Input: dimensioned drawing with shaded views. Units: mm. Origin: part minimum x, y, z. Round coordinates to 2 decimals unless told otherwise and drop trailing zeros. Loops run counter-clockwise (first coordinate to the right, second up) from the corner with the lowest first, then second, coordinate; pieces in that order, holes last. Notation, with made-up numbers: M 21.5,64 L 49.5,64 A21 cw 49.5,101 Z; hole C 65,-36 d9. An arc over 180 degrees is marked long. Write each question's results on one line, items separated by ' | '. Start each with the question number.
1. Section C-C on x = 2.25. Output: boundary loops of the cut face in (y, z), and give its area (3 significant figures).
2. Section B-B on y = 24.5. Output: boundary loops of the cut face in (x, z), and give its area (3 significant figures).
3. Draft query along X for the marked faces 1, 2, 3 and 4. Return one class per face: released by +X, released by -X, zero draft, split by the parting line, or undercut.
4. Contact query for flat-ended pins moving along their axis: pin 1 Ø4 at (x, z) = (17.5, 4) entering from -Y; pin 2 Ø1 at (y, z) = (22.5, 6.5) entering from -X (1 decimal); pin 3 Ø1 at (y, z) = (17, 7.5) entering from -X. Output: stop coordinate, or through.
5. Ray query, line 1 (X direction, y = 12, z = 3.5) (1 decimal); line 2 (Y direction, x = 16.5, z = 7.75) (1 decimal); line 3 (X direction, y = 18, z = 10.75) (1 decimal). Return the intervals inside material, ascending.
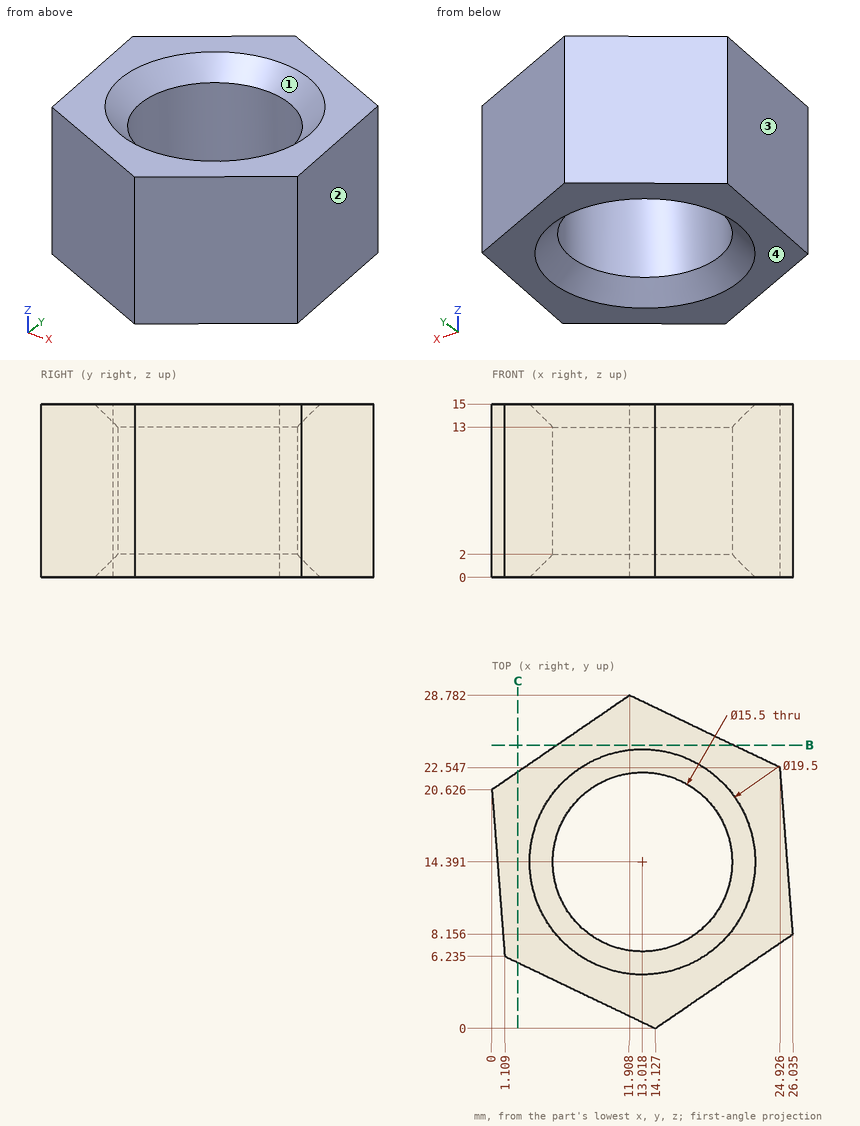
Taken from the geometry:
1) outline: M 5.69,0 L 22.17,0 L 22.17,15 L 5.69,15 Z | area: 247 mm^2
2) outline: M 5.66,0 L 20.85,0 L 20.85,15 L 5.66,15 Z | area: 228 mm^2
3) face 1: undercut | face 2: released by +X | face 3: released by -X | face 4: zero draft
4) pin 1: y = 0.94 | pin 2: x = 2 | pin 3: x = 0.24
5) line 1: 0.7 to 5.6, 20.4 to 25.7 | line 2: 1.6 to 7.5, 21.3 to 26.6 | line 3: 0.2 to 6.2, 19.9 to 25.3
